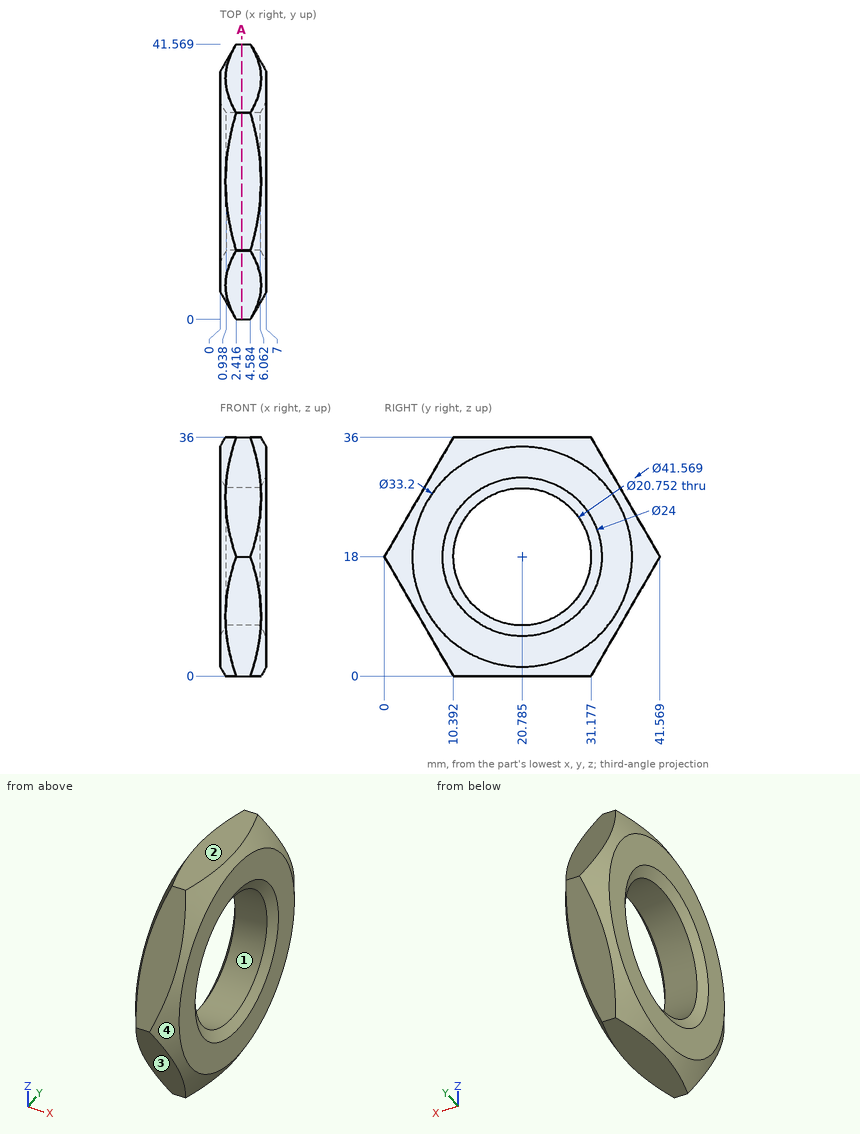
Design review of the part shown in the three views and the two pictorial views. Dimensions are in mm from the part's minimum x, y and z. Give positions to 0.01 mm unless a question says otherwise; leave off trailing zeros. Write each loop counter-clockwise with the first axis right and the second up, starting at its lowest first coordinate (ties: lowest second). Pieces come first, ordered by that corner, then holes. Notation, with made-up numbers: M 81,-21.5 L 92,-21.5 A22 ccw 92,8.5 Z; hole C 25,34.25 d7. An arc over 180 degrees is marked long. Return JSON: item names as keys, results as strings. Group by question number.
Item 1: Wall thickness on line 1 along Y through (x, z) = (2.65, 18); line 2 along Z through (x, y) = (2, 19); line 3 along Z through (x, y) = (4.5, 23.5) (1 decimal): over which ranges is each line inside the solid? List them lowest first.
Item 2: The part is to be moulded in two halves that separate along Y. For the marked faces 1, 2, 3 and 4, say which applies: pulls with the +Y half, pulls with the -Y half, needs draft (parallel to the pull), parting line crosses it, or undercut.
Item 3: Clearance check with flat-ended pins moving along their axes: pin 1 Ø1.5 at (x, z) = (4.5, 13) entering from -Y (1 decimal); pin 2 Ø3 at (x, z) = (4, 4.5) entering from -Y. State where each tip first meets the part, or that it passes through.
Item 4: Take a section at A-A (x = 3.25). Give the boundary of the cut face in (y, z) (1 decimal), plus the area to 3 significant figures.
Return value:
{
 "1": {"line 1": "y = 0 to 10.41, 31.16 to 41.57", "line 2": "z = 0 to 7.78, 28.22 to 36", "line 3": "z = 0 to 8, 28 to 36"},
 "2": {"face 1": "undercut", "face 2": "needs draft", "face 3": "pulls with the -Y half", "face 4": "parting line crosses it"},
 "3": {"pin 1": "stops at y = 2.5", "pin 2": "stops at y = 6.93"},
 "4": {"outline": "M 0,18 L 10.4,0 L 31.2,0 L 41.6,18 L 31.2,36 L 10.4,36 Z; hole C 20.8,18 d20.8", "area": "784 mm2"}
}
